For this review, take the finished solid that the model builds, in its own axes (mm). Face numbers are marked on the shaded views. A direction names the side the tool comes from. Round coordinates to 2 decimals unless told otherwise and drop trailing zeros. Order: outer loops, then holes, each group sorted by start corner. A loop starts at its lowest first (then second) coordinate and runs counter-clockwise, first axis right, second up. Notation, with made-up numbers: (60.5, 18.5) - (102.5, 18.5) arc R20 cw to (102.5, 34.5) - close; hole circle Ø7 at (88, 80.5). An arc over 180 degrees is marked (long way). One line per item, written item: value.
```python
from build123d import *

# Parameters (mm, degrees)
CROQUIS1_W              = 30
CROQUIS1_H              = 20
SALIENTE_EXTRUIR1_DEPTH = 6
CROQUIS3_R              = 1.6
CORTAR_EXTRUIR2_DEPTH   = 40
SALIENTE_EXTRUIR2_START = 2
CROQUIS4_R              = 2.05
CROQUIS4_R_2            = 1.6
SALIENTE_EXTRUIR2_DEPTH = 2
CORTAR_EXTRUIR3_DEPTH   = 3
CROQUIS6_W              = 10
CROQUIS6_H              = 3
CORTAR_EXTRUIR4_DEPTH   = 24
CROQUIS7_R              = 1
CORTAR_EXTRUIR5_DEPTH   = 24
CROQUIS8_W              = 1
CROQUIS8_H              = 3
SALIENTE_EXTRUIR3_DEPTH = 5


with BuildPart() as part:
    # Croquis1 → Saliente-Extruir1 (new body)
    with BuildSketch(Plane(origin=(0, 0, 0), x_dir=(1, 0, 0), z_dir=(0, 1, 0))):
        with Locations((15, 10)):
            Rectangle(CROQUIS1_W, CROQUIS1_H)
    extrude(amount=SALIENTE_EXTRUIR1_DEPTH)

    # Croquis3 → Cortar-Extruir2 (cut)
    with BuildSketch(Plane(origin=(0, 6, 0), x_dir=(1, 0, 0), z_dir=(0, 1, 0))):
        with Locations(Location((6, 5, 0), (0, 0, 270))):
            Circle(CROQUIS3_R)
        with Locations(Location((6, 15, 0), (0, 0, 270))):
            Circle(CROQUIS3_R)
    extrude(amount=-CORTAR_EXTRUIR2_DEPTH, mode=Mode.SUBTRACT)

    # Croquis4 → Saliente-Extruir2 (add)
    # profile 1 of 2: a face of its own
    with BuildSketch(Plane(origin=(0, 6, 0), x_dir=(1, 0, 0), z_dir=(0, 1, 0)).offset(SALIENTE_EXTRUIR2_START)):
        with Locations(Location((6, 15, 0), (0, 0, 90))):
            Circle(CROQUIS4_R)
        with Locations(Location((6, 15, 0), (0, 0, 270))):
            Circle(CROQUIS4_R_2, mode=Mode.SUBTRACT)
    # profile 2 of 2: a face of its own
    with BuildSketch(Plane(origin=(0, 6, 0), x_dir=(1, 0, 0), z_dir=(0, 1, 0)).offset(SALIENTE_EXTRUIR2_START)):
        with Locations(Location((6, 5, 0), (0, 0, 90))):
            Circle(CROQUIS4_R)
        with Locations(Location((6, 5, 0), (0, 0, 270))):
            Circle(CROQUIS4_R_2, mode=Mode.SUBTRACT)
    extrude(amount=-SALIENTE_EXTRUIR2_DEPTH)

    # Croquis5 → Cortar-Extruir3 (cut)
    with BuildSketch(Plane.XZ):
        Polygon((9, -6.732050808), (9, -3.267949192), (6, -1.535898385), (3, -3.267949192), (3, -6.732050808), (6, -8.464101615), align=None)
        Polygon((9, -16.732050808), (9, -13.267949192), (6, -11.535898385), (3, -13.267949192), (3, -16.732050808), (6, -18.464101615), align=None)
    extrude(amount=-CORTAR_EXTRUIR3_DEPTH, mode=Mode.SUBTRACT)

    # Croquis6 → Cortar-Extruir4 (cut)
    with BuildSketch(Plane.XY):
        with Locations((25, 1.5)):
            Rectangle(CROQUIS6_W, CROQUIS6_H)
    extrude(amount=-CORTAR_EXTRUIR4_DEPTH, mode=Mode.SUBTRACT)

    # Croquis7 → Cortar-Extruir5 (cut)
    with BuildSketch(Plane(origin=(0, 6, 0), x_dir=(1, 0, 0), z_dir=(0, 1, 0))):
        with Locations(Location((6, 10, 0), (0, 0, 270))):
            Circle(CROQUIS7_R)
    extrude(amount=-CORTAR_EXTRUIR5_DEPTH, mode=Mode.SUBTRACT)

    # Croquis8 → Saliente-Extruir3 (add)
    with BuildSketch(Plane(origin=(0, 6, 0), x_dir=(1, 0, 0), z_dir=(0, 1, 0))):
        with Locations((7.5, 10)):
            Rectangle(CROQUIS8_W, CROQUIS8_H)
    extrude(amount=SALIENTE_EXTRUIR3_DEPTH)


solid = part.part
```
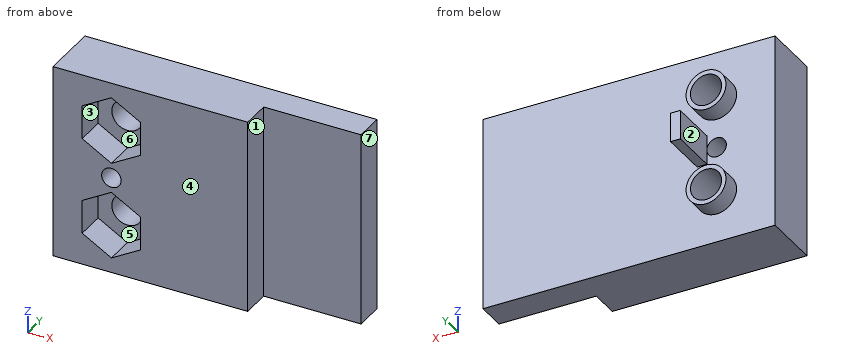
Item 1: The part is to be moulded in two halves that separate along X. For the marked faces 4, 5, 6 and 7, say which applies: +X half, -X half, draft (parallel to the pull), parting line (faces both ways), or undercut.
Returned:
face 4: draft
face 5: undercut
face 6: undercut
face 7: +X half
Item 2: Take a section at C-C (x = 5.5). Count the separate pieces of the cut face and the enclosed holes in it, plus the area to 3 significant figures.
Returned:
separate pieces: 4
enclosed holes: 0
area: 57.0 mm^2
Item 3: Take a section at D-D (x = 19). Write out the cut boundary in (y, z).
Returned:
outline: (0, -20) - (6, -20) - (6, 0) - (0, 0) - close
Item 4: Machinability: for the marked faces 1, 2 and 3, which of the approach directions +Z, -Z, +X, -X, +Y, -Y give a long, thin tool a straight path to every point of the face, cutting with its end or side? Answer none if there is none.
Returned:
face 1: +Z, -Z, +X, -Y
face 2: -X, +Y
face 3: -Y
Item 5: Take a section at B-B (y = 1.75). Write out the cut boundary in (x, z), plus the area to 3 significant figures.
Returned:
outline: (0, -20) - (20, -20) - (20, 0) - (0, 0) - close; hole (3, -16.73) - (6, -18.46) - (9, -16.73) - (9, -13.27) - (6, -11.54) - (3, -13.27) - close; hole (3, -6.73) - (6, -8.46) - (9, -6.73) - (9, -3.27) - (6, -1.54) - (3, -3.27) - close; hole circle Ø2 at (6, -10)
area: 335 mm^2
Item 6: For P1, Ø3, axis at x = 5, y = 8.5, coming from the -Z side; P2, Ø6, axis at x = 16.5, z = -15.5, coming from the +Y side; P3, Ø11, axis at x = 27, z = -5.5, coming from the -Y side, all flat-tipped, find the tip position at first contact; note any pin that passes through.
Returned:
P1: z = -17.05
P2: y = 6
P3: y = 3
Item 7: Take a section at A-A (z = -15). Write out the cut boundary in (x, y).
Returned:
outline: (0, 0) - (3, 0) - (3, 3) - (4.4, 3) - (4.4, 8) - (3.95, 8) - (3.95, 6) - (0, 6) - close; (7.6, 3) - (9, 3) - (9, 0) - (20, 0) - (20, 3) - (30, 3) - (30, 6) - (8.05, 6) - (8.05, 8) - (7.6, 8) - close
Item 8: Wall thickness on line 1 (X direction, y = 7.5, z = -5); line 2 (X direction, y = 4.5, z = -10); line 3 (Y direction, x = 22.25, z = -9.25): over which ranges is each line inside the solid? List them lowest first.
Returned:
line 1: 3.95 to 4.4, 7.6 to 8.05
line 2: 0 to 5, 7 to 30
line 3: 3 to 6
